from build123d import *

# Parameters (mm, degrees)
CROQUIS1_W              = 10
CROQUIS1_H              = 10
SALIENTE_EXTRUIR1_DEPTH = 10
CROQUIS2_R              = 0.5
CORTAR_EXTRUIR1_DEPTH   = 5


with BuildPart() as part:
    # Croquis1 → Saliente-Extruir1 (new body)
    with BuildSketch(Plane(origin=(0, 0, 0), x_dir=(1, 0, 0), z_dir=(0, 1, 0))):
        with Locations((5, 5)):
            Rectangle(CROQUIS1_W, CROQUIS1_H)
    extrude(amount=SALIENTE_EXTRUIR1_DEPTH)

    # Croquis2 → Cortar-Extruir1 (cut)
    with BuildSketch(Plane.XZ):
        with Locations(Location((5, -5, 0), (0, 0, 270))):
            Circle(CROQUIS2_R)
    extrude(amount=-CORTAR_EXTRUIR1_DEPTH, mode=Mode.SUBTRACT)


solid = part.part
Design review of the part built by this model. Coordinates are the model's own, in mm. A direction names the side the tool comes from. Round coordinates to 2 decimals unless told otherwise and drop trailing zeros. Write each loop counter-clockwise with the first axis right and the second up, starting at its lowest first coordinate (ties: lowest second). Pieces come first, ordered by that corner, then holes. Notation, with made-up numbers: (42, 35.5) - (91, 35.5) arc R4 cw to (91, 41.5) - close; hole circle Ø9 at (36.5, 85.25). An arc over 180 degrees is marked (long way). Use a Markdown table: item, result. Add a question column.
1. For faces 4 (the face through (5, 10, -5)), 5 (the face through (5, 5, -5)), list the 3-axis set-ups (+Z, -Z, +X, -X, +Y, -Y) from which the entire face can be reached by the end or side of a thin tool; tool diameter is ignored.
2. Clearance check with a flat-ended pin moving along its axis: pin 1 (4 mm diameter, centred on x = 6.5, y = 3, fed in from +Z). State where the tip first meets the part, or that it passes through.
3. We need section A-A (z = -5). State the section outline as (x, y) points.
4. We need section B-B (x = 5). State the section outline as (y, z) points, then the cut area to 3 significant figures.
5. Wall thickness on probe 1 along X at (y, z) = (3.7, -5): over which ranges is the line inside the solid? List them lowest first.
6. Mouldability with a two-part tool opening along Z and no side actions: class faces 1 (the face through (5, 5, -10)), 2 (the face through (5.496, 2.465, -4.935)), 3 (the face through (6, 0, -5)) as +Z half, -Z half, draft (parallel to the pull), parting line (faces both ways), or undercut.
Output:
| question | item | result |
|---|---|---|
| 1 | face 4 | +Z, -Z, +X, -X, +Y |
| 1 | face 5 | -Y |
| 2 | pin 1 | stops at z = 0 |
| 3 | outline | (0, 0) - (4.5, 0) - (4.5, 5) - (5.5, 5) - (5.5, 0) - (10, 0) - (10, 10) - (0, 10) - close |
| 4 | outline | (0, -10) - (10, -10) - (10, 0) - (0, 0) - (0, -4.5) - (5, -4.5) - (5, -5.5) - (0, -5.5) - close |
| 4 | area | 95.0 mm2 |
| 5 | probe 1 | x = 0 to 4.5, 5.5 to 10 |
| 6 | face 1 | -Z half |
| 6 | face 2 | undercut |
| 6 | face 3 | draft |
